Check sheet for the modelled part. Datum: model origin and axes. Units: mm. A direction names the side the tool comes from. Give positions to 0.01 mm unless a question says otherwise; leave off trailing zeros. Loops run counter-clockwise (first coordinate to the right, second up) from the corner with the lowest first, then second, coordinate; pieces in that order, holes last. Notation, with made-up numbers: (37, -25) - (94, -25) arc R19 cw to (94, 8) - close; hole circle Ø11 at (-16.5, 10.5). An arc over 180 degrees is marked (long way). Use one line per item in the form item = value.
from build123d import *

# Parameters (mm, degrees)
BOSS_EXTRUDE1_DEPTH     = 10
CUT_EXTRUDE2_DEPTH      = 154.297097168
FILLET1_R               = 10
FILLET2_R               = 5
CUT_EXTRUDE3_DEPTH      = 154.297097168
CUT_EXTRUDE3_DEPTH_BACK = 154.297097168
SKETCH3_W               = 7.75
SKETCH3_H               = 5.25
CUT_EXTRUDE6_DEPTH      = 154.297097168
CUT_EXTRUDE6_DEPTH_BACK = 154.297097168
SKETCH6_R               = 1.825
FILLET3_R               = 5
CUT_EXTRUDE7_DEPTH      = 154.297097168
CUT_EXTRUDE7_DEPTH_BACK = 154.297097168
SKETCH7_W               = 35.844648394
SKETCH7_H               = 9.75
SKETCH7_W_2             = 30.675
SKETCH7_H_2             = 5.25
FILLET4_R               = 2.5
SKETCH8_W               = 5
SKETCH8_H               = 5
CUT_EXTRUDE8_DEPTH      = 10
FILLET5_R               = 2
FILLET6_R               = 2
FILLET7_R               = 2
FILLET8_R               = 2


# Some blends are built 0.0001 mm under size
with BuildPart() as part:
    # Sketch1 → Boss-Extrude1 (new body)
    with BuildSketch(Plane(origin=(0, 0, 0), x_dir=(0, 0, -1), z_dir=(1, 0, 0))):
        Polygon((0, 0), (150, 0), (150, 15), (75, 30), (30.773502692, 30), (25, 20), (0, 20), align=None)
    extrude(amount=-BOSS_EXTRUDE1_DEPTH)

    # Sketch2 → Cut-Extrude2 (cut, through all)
    with BuildSketch(Plane(origin=(0, 0, 0), x_dir=(0, 0, -1), z_dir=(1, 0, 0))):
        with BuildLine():
            Line((5, 11.994492417), (5, 8.005507583))
            ThreePointArc((5, 8.005507583), (10.85, 10), (5, 11.994492417))
        make_face()
    extrude(amount=-CUT_EXTRUDE2_DEPTH, mode=Mode.SUBTRACT)

    # Fillet1
    fillet1_edges = [part.edges().sort_by_distance(p)[0] for p in [
        (-5, 0, 0),
        (-5, 20, 0),
    ]]
    fillet(fillet1_edges, radius=FILLET1_R - 0.0001)  # a hair under: the kernel refuses the full size

    # Fillet2
    fillet2_edges = [part.edges().sort_by_distance(p)[0] for p in [
        (-5, 30, -30.773502692),
        (-5, 30, -75),
    ]]
    fillet(fillet2_edges, radius=FILLET2_R)

    # Sketch3 → Cut-Extrude3 (cut, two sides: drawn at the far end of the back side and taken through both)
    with BuildSketch(Plane(origin=(0, 0, 0), x_dir=(0, 0, -1), z_dir=(1, 0, 0)).offset(-CUT_EXTRUDE3_DEPTH_BACK)):
        with Locations((61.125, 7.625)):
            Rectangle(SKETCH3_W, SKETCH3_H)
        with Locations((43.875, 7.625)):
            Rectangle(SKETCH3_W, SKETCH3_H)
    extrude(amount=CUT_EXTRUDE3_DEPTH + CUT_EXTRUDE3_DEPTH_BACK, mode=Mode.SUBTRACT)

    # Sketch6 → Cut-Extrude6 (cut, two sides: drawn at the far end of the back side and taken through both)
    with BuildSketch(Plane(origin=(0, 0, 0), x_dir=(0, 0, -1), z_dir=(1, 0, 0)).offset(-CUT_EXTRUDE6_DEPTH_BACK)):
        with Locations((112.5, 7.5)):
            Circle(SKETCH6_R)
        with Locations((137.5, 7.5)):
            Circle(SKETCH6_R)
    extrude(amount=CUT_EXTRUDE6_DEPTH + CUT_EXTRUDE6_DEPTH_BACK, mode=Mode.SUBTRACT)

    # Fillet3
    fillet3_edges = [part.edges().sort_by_distance(p)[0] for p in [
        (-5, 20, -25),
    ]]
    fillet(fillet3_edges, radius=FILLET3_R)

    # Sketch7 → Cut-Extrude7 (cut, two sides: drawn at the far end of the back side and taken through both)
    with BuildSketch(Plane(origin=(0, 0, 0), x_dir=(0, 0, -1), z_dir=(1, 0, 0)).offset(-CUT_EXTRUDE7_DEPTH_BACK)):
        with Locations((51.582578235, 20.125)):
            Rectangle(SKETCH7_W, SKETCH7_H)
        with Locations((85.3375, 7.625)):
            Rectangle(SKETCH7_W_2, SKETCH7_H_2)
        Polygon((100.675, 15.25), (100.675, 19.765980486), (74.504902432, 25), (74.504902432, 15.25), align=None)
    extrude(amount=CUT_EXTRUDE7_DEPTH + CUT_EXTRUDE7_DEPTH_BACK, mode=Mode.SUBTRACT)

    # Fillet4
    # the kernel refuses this fillet: 2.5 mm, written as the material it adds along each edge
    with BuildSketch(Plane(origin=(0, 15.25, -69.504902432), x_dir=(0, 0, 1), z_dir=(-1, 0, 0)), Plane(origin=(-10, 25, -33.660254038), x_dir=(0, -1, 0), z_dir=(1, 0, 0)), Plane(origin=(0, 25, -69.504902432), x_dir=(0, -1, 0), z_dir=(-1, 0, 0)), Plane(origin=(0, 15.25, -74.504902432), x_dir=(0, 1, 0), z_dir=(-1, 0, 0)), Plane(origin=(0, 15.25, -100.675), x_dir=(0, 0, 1), z_dir=(-1, 0, 0)), Plane(origin=(0, 5, -100.675), x_dir=(0, 0, 1), z_dir=(-1, 0, 0))) as fillet4_piece_1:
        with BuildLine():
            CenterArc((FILLET4_R, FILLET4_R), FILLET4_R, 180, 90)
            Line((0, FILLET4_R), (0, 0))
            Line((0, 0), (FILLET4_R, 0))
        make_face()
    extrude(amount=10)
    with BuildSketch(Plane(origin=(-10, 15.25, -33.660254038), x_dir=(0, 1, 0), z_dir=(1, 0, 0)), Plane(origin=(-10, 5, -70), x_dir=(0, 1, 0), z_dir=(1, 0, 0)), Plane(origin=(-10, 10.25, -70), x_dir=(0, 0, -1), z_dir=(1, 0, 0)), Plane(origin=(0, 10.25, -100.675), x_dir=(0, 0, 1), z_dir=(-1, 0, 0))) as fillet4_piece_2:
        with BuildLine():
            CenterArc((FILLET4_R, -FILLET4_R), FILLET4_R, 90, 90)
            Line((0, -FILLET4_R), (0, 0))
            Line((0, 0), (FILLET4_R, 0))
        make_face()
    extrude(amount=10)
    with BuildSketch(Plane(origin=(-10, 25, -74.504902432), x_dir=(0, -0.1961161351381845, -0.9805806756909201), z_dir=(1, 0, 0))) as fillet4_piece_3:
        with BuildLine():
            CenterArc((FILLET4_R * 1.21980390272, -FILLET4_R), FILLET4_R, 90, 101.309932474)
            Line((FILLET4_R * 0.239223227028, -FILLET4_R * 1.19611613514), (0, 0))
            Line((0, 0), (FILLET4_R * 1.21980390272, 0))
        make_face()
    extrude(amount=10)
    with BuildSketch(Plane(origin=(-10, 19.765980486, -100.675), x_dir=(0, 0.19611613513818169, 0.9805806756909206), z_dir=(1, 0, 0))) as fillet4_piece_4:
        with BuildLine():
            CenterArc((FILLET4_R * 0.819803902719, FILLET4_R), FILLET4_R, 191.309932474, 78.690067526)
            Line((-FILLET4_R * 0.160776772972, FILLET4_R * 0.803883864862), (0, 0))
            Line((0, 0), (FILLET4_R * 0.819803902719, 0))
        make_face()
    extrude(amount=10)

    # Sketch8 → Cut-Extrude8 (cut)
    with BuildSketch(Plane(origin=(0, 0, 0), x_dir=(0, 0, -1), z_dir=(1, 0, 0))):
        with Locations((105.5, 7.5)):
            Rectangle(SKETCH8_W, SKETCH8_H)
    extrude(amount=-CUT_EXTRUDE8_DEPTH, mode=Mode.SUBTRACT)

    # Fillet5
    fillet5_edges = [part.edges().sort_by_distance(p)[0] for p in [
        (0, 7.5, -103),
    ]]
    fillet(fillet5_edges, radius=FILLET5_R)

    # Fillet6
    fillet6_edges = [part.edges().sort_by_distance(p)[0] for p in [
        (-10, 7.5, -108),
    ]]
    fillet(fillet6_edges, radius=FILLET6_R)

    # Fillet7
    fillet7_edges = [part.edges().sort_by_distance(p)[0] for p in [
        (-10, 7.5, -103),
    ]]
    fillet(fillet7_edges, radius=FILLET7_R)

    # Fillet8
    fillet8_edges = [part.edges().sort_by_distance(p)[0] for p in [
        (0, 7.5, -108),
    ]]
    fillet(fillet8_edges, radius=FILLET8_R)


solid = part.part
Item 1: Mould release check, pull along X, two halves, no side actions. Record for faces 1 (the face through (-5, 7, -150)), 2 (the face through (0, 13, -75)): released by +X, released by -X, zero draft, split by the parting line, or undercut.
Answer block:
face_1 = zero draft
face_2 = released by +X
Item 2: Thickness scan on L1, parallel to Y at x = -1.75, z = -61.5; L2, parallel to Y at x = -2.75, z = -48; L3, parallel to Y at x = -6.75, z = -112.5 (3 decimals). Record the ranges inside material, lowest first.
Answer block:
L1 = 0 to 5, 10.25 to 15.25, 25 to 30
L2 = 0 to 15.25, 25 to 30
L3 = 0 to 5.675, 9.325 to 22.5
Item 3: Access from +Z, -Z, +X, -X, +Y, -Y to the whole of each face (thin tool, end or side, straight path). Record for faces 3 (the face through (-5.07, 23.9, -75.44)), 4 (the face through (-5, 30, -54)), 5 (the face through (-5, 20, -16)).
Answer block:
face_3 = +X, -X
face_4 = +Z, -Z, +X, -X, +Y
face_5 = +Z, +X, -X, +Y
Item 4: Section check B-B on x = -6. Give the number of separate pieces and of enclosed holes in the cut face, then the cut area to 3 significant figures.
Answer block:
separate_pieces = 1
enclosed_holes = 9
area = 2,780 mm2
Item 5: Section check C-C on y = 2. Record the boundary of the cut face in (x, z), then the cut area to 3 significant figures.
Answer block:
outline = (-10, -150) - (0, -150) - (0, -4) - (-10, -4) - close
area = 1,460 mm2
Item 6: Section check A-A on z = -112.5. Record the boundary of the cut face in (x, y) (3 decimals).
Answer block:
outline = (-10, 0) - (0, 0) - (0, 5.675) - (-10, 5.675) - close; (-10, 9.325) - (0, 9.325) - (0, 22.5) - (-10, 22.5) - close
Item 7: Gauge pin test, flat ends, axial feed: P1, Ø2.5, axis at x = -5.5, y = 6.5, coming from the +Z side; P2, Ø1.6, axis at x = -5.5, y = 7, coming from the +Z side (3 decimals); P3, Ø2, axis at x = -3, z = -130, coming from the +Y side. Record the tip position at first contact, or that the pin passes through.
Answer block:
P1 = -0.26
P2 = -0.245
P3 = 19.2
